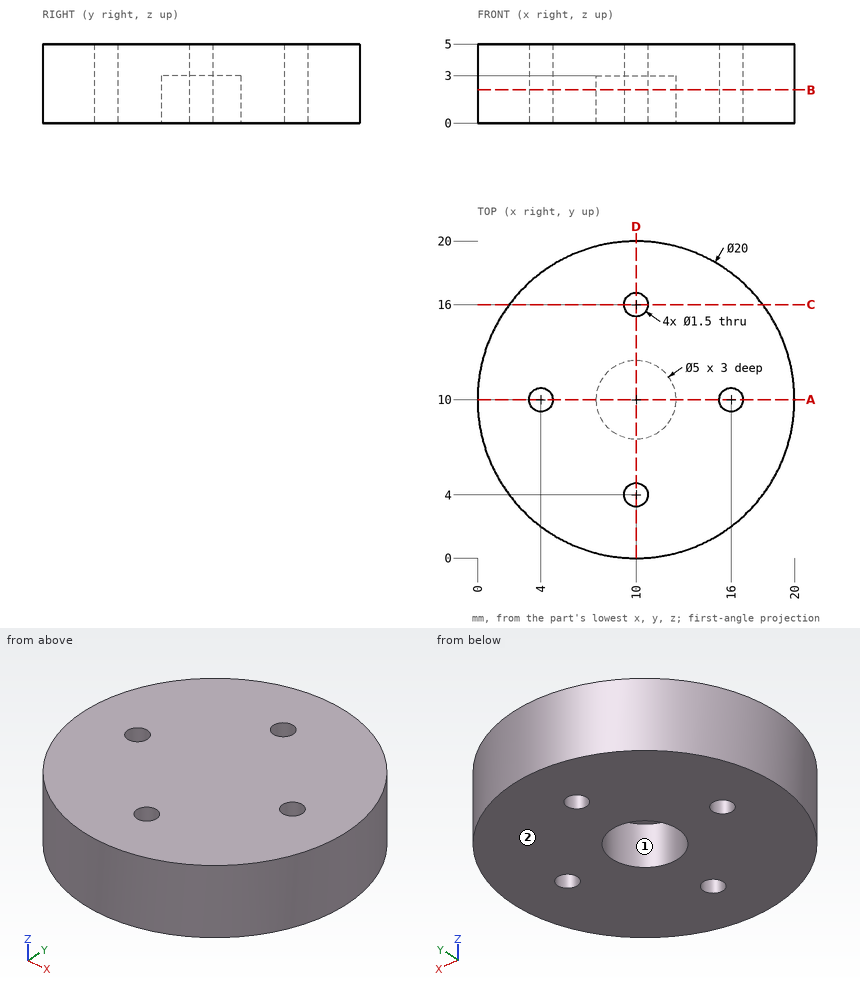
Part print with two shaded views. Sizes in mm from the minimum x, y, z corner. A direction names the side the tool comes from. Round coordinates to 2 decimals unless told otherwise and drop trailing zeros. Order: outer loops, then holes, each group sorted by start corner. A loop starts at its lowest first (then second) coordinate and runs counter-clockwise, first axis right, second up. Notation, with made-up numbers: (-32, 20.5) -> (-21, 20.5) arc R23 cw to (-21, 52.5) -> close; hole circle Ø10 at (51.5, 89.25). An arc over 180 degrees is marked (long way). Use one line per item in the form item = value.
Item 1: Flat gauge pins, fed straight in: pin 1 Ø0.9 at (x, y) = (10, 4) entering from -Z; pin 2 Ø4.5 at (x, y) = (10, 10) entering from -Z. Where does each tip first touch, or does it go through?
Returned:
pin_1 = through
pin_2 = 3
Item 2: Cut at B-B, the plane z = 2.1. Write the cut outline in (x, y).
Returned:
outline = circle Ø20 at (10, 10); hole circle Ø1.5 at (4, 10); hole circle Ø5 at (10, 10); hole circle Ø1.5 at (10, 4); hole circle Ø1.5 at (10, 16); hole circle Ø1.5 at (16, 10)
Item 3: Tool access for the marked faces 1 and 2: list every direction of +Z, -Z, +X, -X, +Y, -Y with a clear straight run to the whole face (end or side of a thin tool).
Returned:
face_1 = -Z
face_2 = -Z, +X, -X, +Y, -Y
Item 4: Drill centre lines: line 1 (Y direction, x = 10, z = 3.6); line 2 (Y direction, x = 10, z = 1.4); line 3 (Y direction, x = 4, z = 2.9). Where is each one in solid material? Low to high.
Returned:
line_1 = 0 to 3.25, 4.75 to 15.25, 16.75 to 20
line_2 = 0 to 3.25, 4.75 to 7.5, 12.5 to 15.25, 16.75 to 20
line_3 = 2 to 9.25, 10.75 to 18
Item 5: Cut at A-A, the plane y = 10. Write the cut outline in (x, z), and give its area (3 significant figures).
Returned:
outline = (0, 0) -> (3.25, 0) -> (3.25, 5) -> (0, 5) -> close; (4.75, 0) -> (7.5, 0) -> (7.5, 3) -> (12.5, 3) -> (12.5, 0) -> (15.25, 0) -> (15.25, 5) -> (4.75, 5) -> close; (16.75, 0) -> (20, 0) -> (20, 5) -> (16.75, 5) -> close
area = 70.0 mm^2
Item 6: Cut at C-C, the plane y = 16. Write the cut outline in (x, z), and give its area (3 significant figures).
Returned:
outline = (2, 0) -> (9.25, 0) -> (9.25, 5) -> (2, 5) -> close; (10.75, 0) -> (18, 0) -> (18, 5) -> (10.75, 5) -> close
area = 72.5 mm^2
